Geometry: final body of the model. Coordinates: model frame, mm. Face numbers are marked on the shaded views. A direction names the side the tool comes from. Give positions to 0.01 mm unless a question says otherwise; leave off trailing zeros. Write each loop counter-clockwise with the first axis right and the second up, starting at its lowest first coordinate (ties: lowest second). Pieces come first, ordered by that corner, then holes.
Q1. Cut plane C-C on y = 105. Return the cut outline in (x, z) (3 decimals), plus the area to 3 significant figures.
Q2. Cut plane D-D on y = -87. Return the cut outline in (x, z), plus the area to 3 significant figures.
Q3. Cut plane A-A on y = 0. Return the cut outline in (x, z), plus the area to 3 significant figures.
Q4. Cut plane B-B on x = -69. Return the cut outline in (y, z).
Q5. Pin query (flat end, axial travel): pin 1 (2 mm diameter, centred on x = -71.5, z = 7.5, fed in from -Y); pin 2 (24 mm diameter, centred on x = -70, y = 0, fed in from -Z); pin 3 (3 mm diameter, centred on x = 33.5, y = 66.5, fed in from -Z); pin 4 (1.5 mm diameter, centred on x = 6.5, y = -6.5, fed in from +Z). Return the tip coordinate at first contact, or that it passes through.
Q6. Line query: L1, parallel to Y at x = -70, z = -6.25; L2, parallel to Z at x = -8, y = -94.5; L3, parallel to X at y = -80.5, z = 0.5. Output: solid intervals per line, ascending.
Q7. Draft query along Y for the marked faces 4 and 5. Return one class per face: pulls with the +Y half, pulls with the -Y half, needs draft (parallel to the pull), parting line crosses it, or undercut.
Q8. Reachability of the marked faces 1, 2 and 3 from +Z, -Z, +X, -X, +Y, -Y: full face, straight path, thin tool, end or side. Return the list, or none.
```python
from build123d import *

# Parameters (mm, degrees)
BOSS_EXTRUDE1_DEPTH = 5
SKETCH1_3_R         = 30
SKETCH1_3_R_2       = 20
SKETCH1_3_R_3       = 25
SKETCH1_3_R_4       = 15
BOSS_EXTRUDE2_DEPTH = 10


with BuildPart() as part:
    # Sketch1 → Boss-Extrude1 (new, symmetric)
    with BuildSketch(Plane.XY):
        with BuildLine():
            ThreePointArc((30, 98), (21.213203436, 76.786796564), (0, 68))
            ThreePointArc((0, 68), (-21.643279891, 77.22577473), (-29.974824802, 99.228770963))
            ThreePointArc((-29.974824802, 99.228770963), (-44.809013245, 56.006438032), (-80.883915711, 27.95604369))
            ThreePointArc((-80.883915711, 27.95604369), (-53.066563718, 24.764061373), (-40, 0))
            ThreePointArc((-40, 0), (-59.649329868, -28.157834217), (-92.857575187, -19.430163575))
            ThreePointArc((-92.857575187, -19.430163575), (-76.859583983, -49.370140698), (-74.716930719, -83.248555502))
            ThreePointArc((-74.716930719, -83.248555502), (-48.118945506, -62.070867765), (-25, -87))
            ThreePointArc((-25, -87), (-28.521882675, -99.794157893), (-38.095238095, -108.983553944))
            ThreePointArc((-38.095238095, -108.983553944), (0, -99.330926563), (38.095238095, -108.983553944))
            ThreePointArc((38.095238095, -108.983553944), (35.626049477, -66.54542725), (74.716930719, -83.248555502))
            ThreePointArc((74.716930719, -83.248555502), (76.859583983, -49.370140698), (92.857575187, -19.430163575))
            ThreePointArc((92.857575187, -19.430163575), (40.914175072, -7.349475372), (80.883915711, 27.95604369))
            ThreePointArc((80.883915711, 27.95604369), (44.809013245, 56.006438032), (29.974824802, 99.228770963))
            ThreePointArc((29.974824802, 99.228770963), (29.99370554, 98.614514416), (30, 98))
        make_face()
    extrude(amount=BOSS_EXTRUDE1_DEPTH, both=True)

    # Sketch1_3 → Boss-Extrude2 (add, symmetric)
    # profile 1 of 8: a face of its own
    with BuildSketch(Plane.XY):
        with BuildLine():
            ThreePointArc((-29.974824802, 99.228770963), (-21.643279891, 77.22577473), (0, 68))
            Line((0, 68), (0, 78))
            ThreePointArc((0, 78), (-20, 98), (0, 118))
            Line((0, 118), (0, 128))
            ThreePointArc((0, 128), (-20.77422527, 119.643279891), (-29.974824802, 99.228770963))
        make_face()
    # profile 2 of 8: a face of its own
    with BuildSketch(Plane.XY):
        with BuildLine():
            Line((0, 78), (0, 68))
            ThreePointArc((0, 68), (21.213203436, 76.786796564), (30, 98))
            ThreePointArc((30, 98), (29.99370554, 98.614514416), (29.974824802, 99.228770963))
            ThreePointArc((29.974824802, 99.228770963), (20.77422527, 119.643279891), (0, 128))
            Line((0, 128), (0, 118))
            ThreePointArc((0, 118), (14.142135624, 112.142135624), (20, 98))
            ThreePointArc((20, 98), (14.142135624, 83.857864376), (0, 78))
        make_face()
    # profile 3 of 8: a face of its own
    with BuildSketch(Plane.XY):
        with BuildLine():
            ThreePointArc((-29.974824802, 99.228770963), (-21.643279891, 77.22577473), (0, 68))
            Line((0, 68), (0, 78))
            ThreePointArc((0, 78), (-20, 98), (0, 118))
            Line((0, 118), (0, 128))
            ThreePointArc((0, 128), (-20.77422527, 119.643279891), (-29.974824802, 99.228770963))
        make_face()
    # profile 4 of 8: a face of its own
    with BuildSketch(Plane.XY):
        with BuildLine():
            Line((0, 78), (0, 68))
            ThreePointArc((0, 68), (21.213203436, 76.786796564), (30, 98))
            ThreePointArc((30, 98), (29.99370554, 98.614514416), (29.974824802, 99.228770963))
            ThreePointArc((29.974824802, 99.228770963), (20.77422527, 119.643279891), (0, 128))
            Line((0, 128), (0, 118))
            ThreePointArc((0, 118), (14.142135624, 112.142135624), (20, 98))
            ThreePointArc((20, 98), (14.142135624, 83.857864376), (0, 78))
        make_face()
    # profile 5 of 8: a face of its own
    with BuildSketch(Plane.XY):
        with Locations((70, 0)):
            Circle(SKETCH1_3_R)
        with Locations((70, 0)):
            Circle(SKETCH1_3_R_2, mode=Mode.SUBTRACT)
    # profile 6 of 8: a face of its own
    with BuildSketch(Plane.XY):
        with Locations((-70, 0)):
            Circle(SKETCH1_3_R)
        with Locations((-70, 0)):
            Circle(SKETCH1_3_R_2, mode=Mode.SUBTRACT)
    # profile 7 of 8: a face of its own
    with BuildSketch(Plane.XY):
        with Locations((-50, -87)):
            Circle(SKETCH1_3_R_3)
        with Locations((-50, -87)):
            Circle(SKETCH1_3_R_4, mode=Mode.SUBTRACT)
    # profile 8 of 8: a face of its own
    with BuildSketch(Plane.XY):
        with Locations((50, -87)):
            Circle(SKETCH1_3_R_3)
        with Locations((50, -87)):
            Circle(SKETCH1_3_R_4, mode=Mode.SUBTRACT)
    extrude(amount=BOSS_EXTRUDE2_DEPTH, both=True)


solid = part.part
```
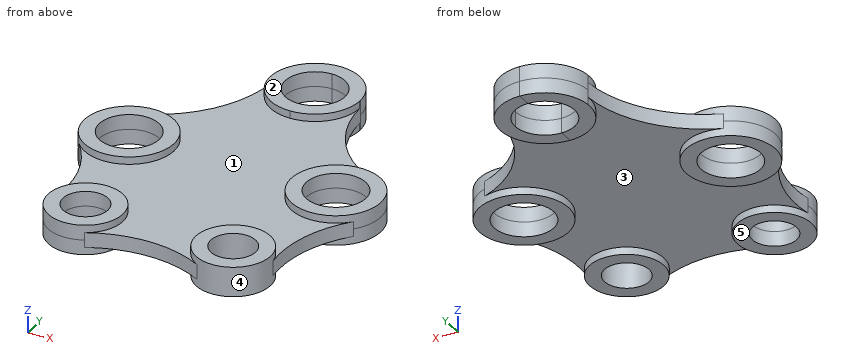
Data:
1. outline: (-29.172, -10) - (-18.735, -10) - (-18.735, 10) - (-29.172, 10) - close; (18.735, -10) - (29.172, -10) - (29.172, 10) - (18.735, 10) - close
1. area: 417 mm2
2. outline: (-75, -10) - (-65, -10) - (-65, 10) - (-75, 10) - close; (-35, -10) - (-25, -10) - (-25, -5) - (25, -5) - (25, -10) - (35, -10) - (35, 10) - (25, 10) - (25, 5) - (-25, 5) - (-25, 10) - (-35, 10) - close; (65, -10) - (75, -10) - (75, 10) - (65, 10) - close
2. area: 1,300 mm2
3. outline: (-100, -10) - (-90, -10) - (-90, 10) - (-100, 10) - close; (-50, -10) - (-40, -10) - (-40, -5) - (40, -5) - (40, -10) - (50, -10) - (50, 10) - (40, 10) - (40, 5) - (-40, 5) - (-40, 10) - (-50, 10) - close; (90, -10) - (100, -10) - (100, 10) - (90, 10) - close
3. area: 1,600 mm2
4. outline: (-103.25, -10) - (-70.75, -10) - (-70.75, -5) - (-29.98, -5) - (-29.98, -10) - (-19.97, -10) - (-19.97, 10) - (-29.98, 10) - (-29.98, 5) - (-70.75, 5) - (-70.75, 10) - (-103.25, 10) - close; (19.97, -10) - (29.98, -10) - (29.98, -5) - (33.76, -5) - (33.76, 5) - (29.98, 5) - (29.98, 10) - (19.97, 10) - close
5. pin 1: stops at y = -101.31
5. pin 2: passes through
5. pin 3: stops at z = -5
5. pin 4: stops at z = 5
6. L1: y = -102 to -72, -30 to -20, 20 to 30
6. L2: z = -5 to 5
6. L3: x = -74.35 to -63.52, -36.48 to 36.48, 63.52 to 74.35
7. face 4: undercut
7. face 5: needs draft
8. face 1: +Z
8. face 2: +Z, +X, -X, +Y, -Y
8. face 3: -Z
